Work out the finished part from the listing and answer in its coordinate system (mm). Coordinates: 2 decimals unless noted, no trailing zeros. Loops run counter-clockwise (first coordinate to the right, second up) from the corner with the lowest first, then second, coordinate; pieces in that order, holes last.
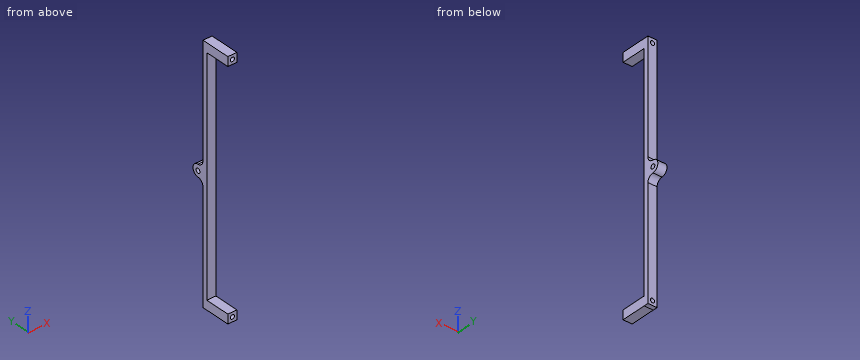
```python
from build123d import *
from build123d.topology import SkipClean

# Parameters (mm, degrees)
SKETCH_1_W      = 10
SKETCH_1_H      = 270
SKETCH_1_R      = 2.25
EXTRUDE_1_DEPTH = 5
SKETCH_2_R      = 2.5
EXTRUDE_2_DEPTH = 10
EXTRUDE_START   = 27.65
SKETCH_3_W      = 10
SKETCH_3_H      = 10
SKETCH_3_R      = 2.25
EXTRUDE_3_DEPTH = 27.65


with BuildPart() as part:
    # Эскиз1 → Бобышка-Вытянуть1 (new body)
    with BuildSketch(Plane(origin=(0, 0, 0), x_dir=(1, 0, 0), z_dir=(0, 1, 0))):
        with Locations((5, 135)):
            Rectangle(SKETCH_1_W, SKETCH_1_H)
        with Locations(Location((5, 265, 0), (0, 0, 270))):
            Circle(SKETCH_1_R, mode=Mode.SUBTRACT)
        with Locations(Location((5, 5, 0), (0, 0, 270))):
            Circle(SKETCH_1_R, mode=Mode.SUBTRACT)
    extrude(amount=EXTRUDE_1_DEPTH)

    # Эскиз2 → Бобышка-Вытянуть2 (add)
    with BuildSketch(Plane(origin=(0, 0, 0), x_dir=(0, 0, -1), z_dir=(1, 0, 0))):
        with BuildLine():
            Line((122, 5), (148, 5))
            ThreePointArc((148, 5), (143.403805922, 6.903805922), (141.5, 11.5))
            ThreePointArc((141.5, 11.5), (135, 18), (128.5, 11.5))
            ThreePointArc((128.5, 11.5), (126.596194078, 6.903805922), (122, 5))
        make_face()
        with Locations((135, 11.5)):
            Circle(SKETCH_2_R, mode=Mode.SUBTRACT)
    extrude(amount=EXTRUDE_2_DEPTH)

    # Эскиз3 → Бобышка-Вытянуть3 (add)
    # profile 1 of 2: a face of its own
    with SkipClean():  # the faces are left unmerged after this step: merging them gives an invalid solid
        with BuildSketch(Plane.XZ.offset(EXTRUDE_START)):
            with Locations((5, -5)):
                Rectangle(SKETCH_3_W, SKETCH_3_H)
            with Locations(Location((5, -5, 0), (0, 0, 90))):
                Circle(SKETCH_3_R, mode=Mode.SUBTRACT)
        # profile 2 of 2: a face of its own
        with BuildSketch(Plane.XZ.offset(EXTRUDE_START)):
            with Locations((5, -265)):
                Rectangle(SKETCH_3_W, SKETCH_3_H)
            with Locations((5, -265)):
                Circle(SKETCH_3_R, mode=Mode.SUBTRACT)
        extrude(amount=-EXTRUDE_3_DEPTH)


solid = part.part
```
1. A cutting plane is placed at D-D, the plane z = -135. Give the vertices of the cut face in (x, y), then the cut area to 3 significant figures.
2. A cutting plane is placed at C-C, the plane z = -5. Give the vertices of the cut face in (x, y), then the cut area to 3 significant figures.
3. Straight lines are drawn through the part: probe 1 along Z at (x, y) = (5, -18); probe 2 along Z at (x, y) = (9, -13.5); probe 3 along Z at (x, y) = (3.5, -6). For each, find the intervals that lie inside material, in ascending order.
4. Each of these flat-tipped pins is pushed along its axis until it touches: P1, Ø6, axis at x = 7.5, y = -6, coming from the +Z side; P2, Ø2, axis at x = 4, y = 11.5, coming from the -Z side; P3, Ø1, axis at x = 6.5, z = -37, coming from the +Y side; P4, Ø5, axis at x = 4, z = -157, coming from the -Y side. Where does it stop, or does it pass through?
5. A cutting plane is placed at B-B, the plane y = -18.5. Give the vertices of the cut face in (x, z), then the cut area to 3 significant figures.
6. A cutting plane is placed at A-A, the plane x = 5. Give the vertices of the cut face in (y, z).
Answers below:
1. outline: (0, 0) - (10, 0) - (10, 9) - (0, 9) - close; (0, 14) - (10, 14) - (10, 18) - (0, 18) - close
1. area: 130 mm2
2. outline: (0, -27.65) - (2.75, -27.65) - (2.75, 5) - (0, 5) - close; (7.25, -27.65) - (10, -27.65) - (10, 5) - (7.25, 5) - close
2. area: 180 mm2
3. probe 1: z = -270 to -267.25, -262.75 to -260, -10 to -7.25, -2.75 to 0
3. probe 2: z = -270 to -260, -10 to 0
3. probe 3: z = -270 to -266.68, -263.32 to -260, -10 to -6.68, -3.32 to 0
4. P1: stops at z = 0
4. P2: stops at z = -141.58
4. P3: stops at y = 5
4. P4: stops at y = 0
5. outline: (0, -270) - (10, -270) - (10, -260) - (0, -260) - close; (0, -10) - (10, -10) - (10, 0) - (0, 0) - close; hole circle Ø4.5 at (5, -265); hole circle Ø4.5 at (5, -5)
5. area: 168 mm2
6. outline: (-27.65, -270) - (5, -270) - (5, -267.25) - (-27.65, -267.25) - close; (-27.65, -262.75) - (5, -262.75) - (5, -148) arc R6.5 cw to (11.5, -141.5) arc R6.5 ccw to (11.5, -128.5) arc R6.5 cw to (5, -122) - (5, -7.25) - (-27.65, -7.25) - (-27.65, -10) - (0, -10) - (0, -260) - (-27.65, -260) - close; (-27.65, -2.75) - (5, -2.75) - (5, 0) - (-27.65, 0) - close; hole circle Ø5 at (11.5, -135)
